CAD build for the part. Positions are in the model's coordinates, mm. Round coordinates to 2 decimals unless told otherwise and drop trailing zeros. Order: outer loops, then holes, each group sorted by start corner. A loop starts at its lowest first (then second) coordinate and runs counter-clockwise, first axis right, second up. Notation, with made-up numbers: M 18,3.25 L 50,3.25 A21 ccw 50,28.25 Z; hole C 25,32.5 d7. An arc over 180 degrees is marked long. Answer as a JSON object with one key per item and string values.
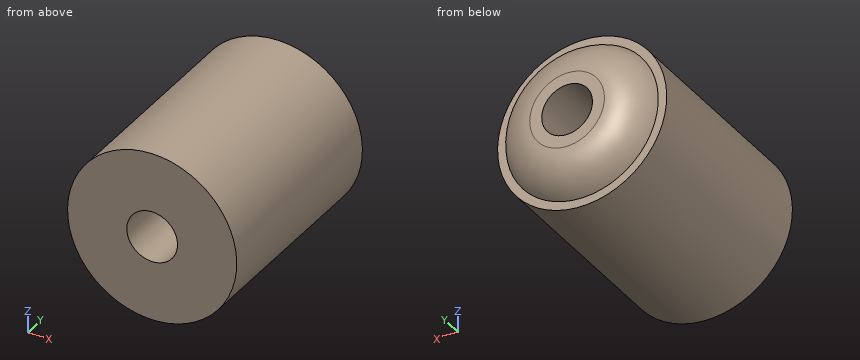
```python
from build123d import *

# Parameters (mm, degrees)
SKETCH1_R           = 10
BOSS_EXTRUDE2_DEPTH = 25
SKETCH2_R           = 9
BOSS_EXTRUDE3_DEPTH = 28
SKETCH3_R           = 3
CUT_EXTRUDE1_DEPTH  = 42
FILLET2_R           = 5


with BuildPart() as part:
    # Sketch1 → Boss-Extrude2 (new body)
    with BuildSketch(Plane(origin=(0, 0, 0), x_dir=(1, 0, 0), z_dir=(0, 1, 0))):
        with Locations(Location((0, 0, 0), (0, 0, 270))):
            Circle(SKETCH1_R)
    extrude(amount=BOSS_EXTRUDE2_DEPTH)

    # Sketch2 → Boss-Extrude3 (add)
    with BuildSketch(Plane(origin=(0, 0, 0), x_dir=(1, 0, 0), z_dir=(0, 1, 0))):
        with Locations(Location((0, 0, 0), (0, 0, 270))):
            Circle(SKETCH2_R)
    extrude(amount=BOSS_EXTRUDE3_DEPTH)

    # Sketch3 → Cut-Extrude1 (cut)
    with BuildSketch(Plane(origin=(0, 0, 0), x_dir=(1, 0, 0), z_dir=(0, 1, 0))):
        with Locations(Location((0, 0, 0), (0, 0, 270))):
            Circle(SKETCH3_R)
    extrude(amount=CUT_EXTRUDE1_DEPTH, mode=Mode.SUBTRACT)

    # Fillet2
    # the kernel refuses this fillet: 5 mm, written as the material it takes off along each edge
    with BuildSketch(Plane(origin=(0, 28, 0), x_dir=(0, 0, 1), z_dir=(-1, 0, 0))) as fillet2_piece_1:
        with BuildLine():
            CenterArc((4.417424305, -5), FILLET2_R, 23.578178478, 66.421821522)
            Line((4.417424305, 0), (4.417424305, 0.1))
            Line((4.417424305, 0.1), (9, 0.1))
            Line((9, 0.1), (9.1, 0))
            ThreePointArc((9.1, 0), (9.1, -1.5), (9.091651514, -2.96))
            Line((9.091651514, -2.96), (9, -3))
        make_face()
    revolve(axis=Axis((0, 28, 0), (0, 1, 0)), mode=Mode.SUBTRACT)


solid = part.part
```
Item 1: Saw through at A-A on y = 18.75. List the corners of the cut face in (x, z), and give its area (3 significant figures).
Worked answers:
{"outline": "C 0,0 d20; hole C 0,0 d6", "area": "286 mm2"}
Item 2: Drop flat-ended pins along their axis: pin 1 Ø10 at (y, z) = (5, -6.5) entering from -X; pin 2 Ø2 at (x, y) = (-3, 9.5) entering from -Z; pin 3 Ø1.5 at (y, z) = (21, -3) entering from -X. Give the stop position or say it passes through.
Worked answers:
{"pin 1": "stops at x = -9.89", "pin 2": "stops at z = -9.8", "pin 3": "stops at x = -9.74"}
Item 3: Wall check: line 1 along X through (y, z) = (6.25, 0); line 2 along Z through (x, y) = (-1.75, 9.75); line 3 along X through (y, z) = (20.75, -9). Give the ranges that are in metal, low to high. Write a range as [from, to].
Worked answers:
{"line 1": "x = [-10, -3], [3, 10]", "line 2": "z = [-9.85, -2.44], [2.44, 9.85]", "line 3": "x = [-4.36, 4.36]"}
